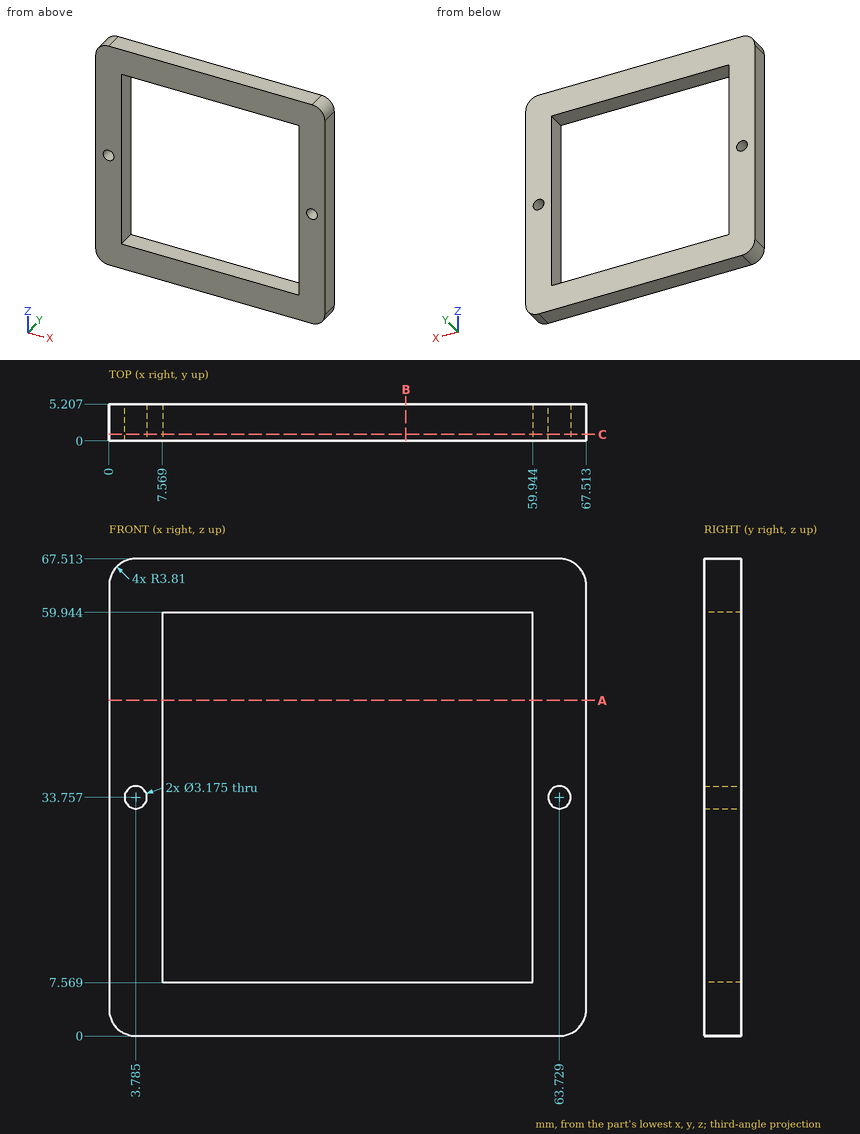
Part print with two shaded views. Sizes in mm from the minimum x, y, z corner. Round coordinates to 2 decimals unless told otherwise and drop trailing zeros. Loops run counter-clockwise (first coordinate to the right, second up) from the corner with the lowest first, then second, coordinate; pieces in that order, holes last. Notation, with made-up numbers: M -33,-32 L 10,-32 A27 cw 10,-1 Z; hole C -15,52.25 d3. An arc over 180 degrees is marked long. Return JSON: item names as keys, results as strings. Group by question number.
(1) Saw through at C-C, the plane y = 0.9. List the corners of the cut face in (x, z) (1 decimal), and give its area (3 significant figures).
(2) Drop flat-ended pins along their axis: P1, Ø5, axis at x = 3.78, z = 33.76, coming from the -Y side; P2, Ø2.5, axis at x = 63.73, z = 33.76, coming from the -Y side. Give the stop position or say it passes through.
(3) Wall check: probe 1 along Z at (x, y) = (24.5, 1.85); probe 2 along X at (y, z) = (0.85, 33.5) (1 decimal). Give the ranges that are in metal, low to high. Write a range as [from, to].
(4) Saw through at B-B, the plane x = 42. List the corners of the cut face in (y, z).
(5) Saw through at A-A, the plane z = 47.5. List the corners of the cut face in (x, y).
Answer list:
{
 "1": {"outline": "M 0,3.8 A3.8 ccw 3.8,0 L 63.7,0 A3.8 ccw 67.5,3.8 L 67.5,63.7 A3.8 ccw 63.7,67.5 L 3.8,67.5 A3.8 ccw 0,63.7 Z; hole C 3.8,33.8 d3.2; hole M 7.6,7.6 L 59.9,7.6 L 59.9,59.9 L 7.6,59.9 Z; hole C 63.7,33.8 d3.2", "area": "1,790 mm2"},
 "2": {"P1": "y = 0", "P2": "through"},
 "3": {"probe 1": "[0, 7.57], [59.94, 67.51]", "probe 2": "[0, 2.2], [5.4, 7.6], [59.9, 62.2], [65.3, 67.5]"},
 "4": {"outline": "M 0,0 L 5.21,0 L 5.21,7.57 L 0,7.57 Z; M 0,59.94 L 5.21,59.94 L 5.21,67.51 L 0,67.51 Z"},
 "5": {"outline": "M 0,0 L 7.57,0 L 7.57,5.21 L 0,5.21 Z; M 59.94,0 L 67.51,0 L 67.51,5.21 L 59.94,5.21 Z"}
}
